```python
from build123d import *

# Parameters (mm, degrees)
SALIENTE_EXTRUIR1_DEPTH = 3
CORTAR_EXTRUIR1_DEPTH   = 102
SALIENTE_EXTRUIR2_DEPTH = 98
CORTAR_EXTRUIR2_DEPTH   = 23
CORTAR_EXTRUIR3_START   = -75
CORTAR_EXTRUIR3_DEPTH   = 23
CHAFL_N1_SIZE           = 2
CROQUIS3_R              = 1.1
CORTAR_EXTRUIR4_DEPTH   = 23
CROQUIS5_R              = 1.75
CORTAR_EXTRUIR5_DEPTH   = 52
CROQUIS6_R              = 1.624451876
CORTAR_EXTRUIR6_DEPTH   = 4
CROQUIS7_R              = 1.624451876
CORTAR_EXTRUIR7_DEPTH   = 4
CROQUIS8_W              = 8
CROQUIS8_H              = 6
CORTAR_EXTRUIR8_DEPTH   = 4


with BuildPart() as part:
    # Croquis1 → Saliente-Extruir1 (new body)
    with BuildSketch(Plane(origin=(0, 0, 0), x_dir=(1, 0, 0), z_dir=(0, 1, 0))):
        Polygon((51.111271676, 38.095375723), (-46.888728324, 38.095375723), (-46.888728324, -36.904624277), (-23.888728324, -36.904624277), (-23.888728324, -54.904624277), (28.111271676, -54.904624277), (28.111271676, -36.904624277), (51.111271676, -36.904624277), align=None)
    extrude(amount=SALIENTE_EXTRUIR1_DEPTH)

    # Croquis2 → Cortar-Extruir1 (cut)
    with BuildSketch(Plane.ZY.offset(46.888728324)):
        Polygon((-38.095375723, 3), (-38.095375723, 0), (-23.398437266, 3), align=None)
    extrude(amount=-CORTAR_EXTRUIR1_DEPTH, mode=Mode.SUBTRACT)

    # Croquis2<4> → Saliente-Extruir2 (add)
    with BuildSketch(Plane.ZY.offset(46.888728324)):
        with BuildLine():
            Line((36.904624277, 1.635706113), (36.904624277, 0))
            Line((36.904624277, 0), (38.738229724, 0))
            ThreePointArc((38.738229724, 0), (37.784681493, 0.776661817), (36.904624277, 1.635706113))
        make_face()
    extrude(amount=-SALIENTE_EXTRUIR2_DEPTH)

    # Croquis2<5> → Cortar-Extruir2 (cut)
    with BuildSketch(Plane.ZY.offset(46.888728324)):
        with BuildLine():
            ThreePointArc((35.783023673, 3), (36.321816168, 2.299760203), (36.904624277, 1.635706113))
            Line((36.904624277, 1.635706113), (36.904624277, 2.693376137))
            ThreePointArc((36.904624277, 2.693376137), (36.779988068, 2.845753154), (36.657673511, 3))
            Line((36.657673511, 3), (35.783023673, 3))
        make_face()
        with BuildLine():
            ThreePointArc((36.657673511, 3), (36.779988068, 2.845753154), (36.904624277, 2.693376137))
            Line((36.904624277, 2.693376137), (36.904624277, 3))
            Line((36.904624277, 3), (36.657673511, 3))
        make_face()
    extrude(amount=-CORTAR_EXTRUIR2_DEPTH, mode=Mode.SUBTRACT)

    # Croquis2<6> → Cortar-Extruir3 (cut)
    with BuildSketch(Plane.ZY.offset(46.888728324).offset(CORTAR_EXTRUIR3_START)):
        with BuildLine():
            ThreePointArc((35.783023673, 3), (36.321816168, 2.299760203), (36.904624277, 1.635706113))
            Line((36.904624277, 1.635706113), (36.904624277, 2.693376137))
            ThreePointArc((36.904624277, 2.693376137), (36.779988068, 2.845753154), (36.657673511, 3))
            Line((36.657673511, 3), (35.783023673, 3))
        make_face()
        with BuildLine():
            ThreePointArc((36.657673511, 3), (36.779988068, 2.845753154), (36.904624277, 2.693376137))
            Line((36.904624277, 2.693376137), (36.904624277, 3))
            Line((36.904624277, 3), (36.657673511, 3))
        make_face()
    extrude(amount=-CORTAR_EXTRUIR3_DEPTH, mode=Mode.SUBTRACT)

    # Chaflán1
    chafl_n1_edges = [part.edges().sort_by_distance(p)[0] for p in [
        (2.111271676, 0, 54.904624277),
    ]]
    chamfer(chafl_n1_edges, length=CHAFL_N1_SIZE)

    # Croquis3 → Cortar-Extruir4 (cut)
    with BuildSketch(Plane(origin=(0, 3, 0), x_dir=(1, 0, 0), z_dir=(0, 1, 0))):
        with Locations(Location((-43.888728324, 3.398437266, 0), (0, 0, 270))):
            Circle(CROQUIS3_R)
        with Locations(Location((-43.888728324, -32.783023673, 0), (0, 0, 270))):
            Circle(CROQUIS3_R)
        with Locations(Location((48.111271676, -32.783023673, 0), (0, 0, 270))):
            Circle(CROQUIS3_R)
        with Locations(Location((48.111271676, 3.398437266, 0), (0, 0, 270))):
            Circle(CROQUIS3_R)
    extrude(amount=-CORTAR_EXTRUIR4_DEPTH, mode=Mode.SUBTRACT)

    # Croquis5 → Cortar-Extruir5 (cut)
    with BuildSketch(Plane(origin=(0, 3, 0), x_dir=(1, 0, 0), z_dir=(0, 1, 0))):
        with Locations(Location((-16.888728324, -38.081562734, 0), (0, 0, 270))):
            Circle(CROQUIS5_R)
        with Locations(Location((21.111271676, -38.081562734, 0), (0, 0, 270))):
            Circle(CROQUIS5_R)
    extrude(amount=-CORTAR_EXTRUIR5_DEPTH, mode=Mode.SUBTRACT)

    # Croquis6 → Cortar-Extruir6 (cut)
    with BuildSketch(Plane(origin=(0, 3, 0), x_dir=(1, 0, 0), z_dir=(0, 1, 0))):
        with Locations(Location((47.381271676, -25.781562734, 0), (0, 0, 270))):
            Circle(CROQUIS6_R)
    extrude(amount=-CORTAR_EXTRUIR6_DEPTH, mode=Mode.SUBTRACT)

    # Croquis7 → Cortar-Extruir7 (cut)
    with BuildSketch(Plane(origin=(0, 3, 0), x_dir=(1, 0, 0), z_dir=(0, 1, 0))):
        with Locations(Location((-43.158728324, -25.781562734, 0), (0, 0, 270))):
            Circle(CROQUIS7_R)
    extrude(amount=-CORTAR_EXTRUIR7_DEPTH, mode=Mode.SUBTRACT)

    # Croquis8 → Cortar-Extruir8 (cut)
    with BuildSketch(Plane(origin=(0, 3, 0), x_dir=(1, 0, 0), z_dir=(0, 1, 0))):
        with Locations((-30.432234651, 12.05730105)):
            Rectangle(CROQUIS8_W, CROQUIS8_H)
        with Locations((34.654778004, 12.05730105)):
            Rectangle(CROQUIS8_W, CROQUIS8_H)
    extrude(amount=-CORTAR_EXTRUIR8_DEPTH, mode=Mode.SUBTRACT)


solid = part.part
```
Check sheet for the modelled part. Datum: model origin and axes. Units: mm. A direction names the side the tool comes from. Round coordinates to 2 decimals unless told otherwise and drop trailing zeros. Order: outer loops, then holes, each group sorted by start corner. A loop starts at its lowest first (then second) coordinate and runs counter-clockwise, first axis right, second up.
1) Tool access check on faces 4 (the flat face through (51.111, 1, 1)), 5 (the flat face through (-30, 2, -9.057)). Record the directions out of +Z, -Z, +X, -X, +Y, -Y that give a thin tool (end or side, any length) a straight path to the whole face; none if there is none.
2) Scan lines: line 1 (X direction, y = 0.65, z = -4); line 2 (X direction, y = 0.5, z = 39); line 3 (X direction, y = 0.6, z = 44). Record each from-to range of solid material in increasing order.
3) Section check C-C (x = -13). Record the boundary of the cut face in (y, z), and give its area (3 significant figures).
4) Section check A-A (x = -30.5). Record the boundary of the cut face in (y, z), and give its area (3 significant figures).
5) Section check D-D (y = 1.05). Give the number of separate pieces and of enclosed holes in the cut face, and give its area (3 significant figures).
6) Mould release check, pull along Z, two halves, no side actions. Record for faces 1 (the cylindrical face through (48.751, 1.521, 26.655)), 2 (the flat face through (-46.889, 2, 0)), 3 (the flat face through (1.43, 1.48, -30.85)): +Z half, -Z half, draft (parallel to the pull), parting line (faces both ways), or undercut.
7) Go/stop test with a flat-tipped pin: pin 1 Ø1.5 at (x, y) = (35.5, 1) entering from +Z. Record where the tip stops, or that it passes through.
8) Section check B-B (z = -13). Record the boundary of the cut face in (x, y).
Result:
1. face 4: +Z, -Z, +X, +Y, -Y
1. face 5: +Y, -Y
2. line 1: x = -46.89 to -44.81, -42.97 to 47.19, 49.03 to 51.11
2. line 2: x = -23.89 to -18.38, -15.4 to 19.62, 22.6 to 28.11
2. line 3: x = -23.89 to 28.11
3. outline: (0, -38.1) - (3, -23.4) - (3, 54.9) - (2, 54.9) - (0, 52.9) - close
3. area: 255 mm2
4. outline: (0, -38.1) - (3, -23.4) - (3, -15.06) - (0, -15.06) - close; (0, -9.06) - (3, -9.06) - (3, 35.78) arc R13.7 cw to (0, 38.74) - close
4. area: 186 mm2
5. separate pieces: 1
5. enclosed holes: 10
5. area: 7,610 mm2
6. face 1: undercut
6. face 2: draft
6. face 3: -Z half
7. pin 1: stops at z = 38.41
8. outline: (-46.89, 0) - (-34.43, 0) - (-34.43, 3) - (-46.89, 3) - close; (-26.43, 0) - (30.65, 0) - (30.65, 3) - (-26.43, 3) - close; (38.65, 0) - (51.11, 0) - (51.11, 3) - (38.65, 3) - close
